```python
from build123d import *

# Parameters (mm, degrees)
CYLINDER001_R     = 4.5
CYLINDER001_DEPTH = 15
CYLINDER_R        = 5
CYLINDER_DEPTH    = 15


with BuildPart() as obj1:
    # Cylinder001 → Cylinder001 (new body)
    with BuildSketch(Plane.XY):
        Circle(CYLINDER001_R)
    extrude(amount=CYLINDER001_DEPTH)


with BuildPart() as cilindro:
    # Cylinder → Cylinder (new body)
    with BuildSketch(Plane.XY):
        Circle(CYLINDER_R)
    extrude(amount=CYLINDER_DEPTH)

    # Cut: cut obj1
    add(obj1.part, mode=Mode.SUBTRACT)


with BuildPart() as cono_interior:
    # Cone001 → Cone001 (revolve)
    with BuildSketch(Plane.XZ):
        Polygon((0, 0), (4.5, 0), (24.5, 30), (0, 30), align=None)
    revolve(axis=Axis((0, 0, 0), (0, 0, 1)))


with BuildPart() as obj2:
    # Cone → Cone (revolve)
    with BuildSketch(Plane.XZ):
        Polygon((0, 0), (5, 0), (25, 30), (0, 30), align=None)
    revolve(axis=Axis((0, 0, 0), (0, 0, 1)))

    # Cut001: cut cono_interior
    add(cono_interior.part, mode=Mode.SUBTRACT)


with BuildPart() as obj2_1:
    # Cut001 placement: moved
    add(obj2.part.moved(Location((0, 0, 15))))

    # Fusion: union cilindro
    add(cilindro.part)


solid = obj2_1.part
```
Geometry check sheet. Reference: the model listing, model coordinates, mm. Round coordinates to 2 decimals unless told otherwise and drop trailing zeros. Loops run counter-clockwise (first coordinate to the right, second up) from the corner with the lowest first, then second, coordinate; pieces in that order, holes last. Notation, with made-up numbers: (65.5, -5.75) - (106.5, -5.75) arc R7 cw to (106.5, 0.25) - close; hole circle Ø9 at (-15, 50.25). An arc over 180 degrees is marked (long way). Use a Markdown table: item, result.
Q1. Draft check along Y on faces 1 (the conical face through (9.725, 3.062, 23.543)), 2 (the cylindrical face through (-1.08, -4.88, 7.4)), 3 (the cylindrical face through (-0.59, 4.46, 7.4)), 4 (the flat face through (18, -17, 45)). Enter one of: released by +Y, released by -Y, zero draft, split by the parting line, or undercut.
Solutions:
| item | result |
|---|---|
| face 1 | undercut |
| face 2 | split by the parting line |
| face 3 | undercut |
| face 4 | zero draft |
Q2. Material ranges on line 1 (Y direction, x = 0, z = 10); line 2 (X direction, y = 18, z = 39); line 3 (X direction, y = 3.5, z = 40.5), recorded low to high.
Solutions:
| item | result |
|---|---|
| line 1 | y = -5 to -4.5, 4.5 to 5 |
| line 2 | x = -10.82 to -9.81, 9.81 to 10.82 |
| line 3 | x = -21.72 to -21.21, 21.21 to 21.72 |
Q3. Go/stop test with flat-tipped pins: P1, Ø2, axis at y = -10.5, z = 37.5, coming from the -X side; P2, Ø1, axis at x = -14, y = -2.5, coming from the -Z side; P3, Ø8, axis at x = -9.5, z = 31, coming from the -Y side. Record where each tip stops, or that it passes through.
Solutions:
| item | result |
|---|---|
| P1 | stops at x = -17.99 |
| P2 | stops at z = 28.08 |
| P3 | stops at y = -16.34 |
Q4. Cross-section at A-A on x = 0. Record the cut outline in (y, z), plus the area to 3 significant figures.
Solutions:
| item | result |
|---|---|
| outline | (-25, 45) - (-5, 15) - (-5, 0) - (-4.5, 0) - (-4.5, 15) - (-24.5, 45) - close; (4.5, 0) - (5, 0) - (5, 15) - (25, 45) - (24.5, 45) - (4.5, 15) - close |
| area | 45.0 mm2 |
Q5. Cross-section at C-C on z = 5.5. Record the cut outline in (x, y).
Solutions:
| item | result |
|---|---|
| outline | circle Ø10 at (0, 0); hole circle Ø9 at (0, 0) |
